For this review, take the finished solid that the model builds, in its own axes (mm). Give positions to 0.01 mm unless a question says otherwise; leave off trailing zeros. Loops run counter-clockwise (first coordinate to the right, second up) from the corner with the lowest first, then second, coordinate; pieces in that order, holes last. Notation, with made-up numbers: (45.25, -16) - (67.25, -16) arc R20 ccw to (67.25, 3) - close; hole circle Ø6 at (-38, 59). An arc over 180 degrees is marked (long way). Answer in a Markdown table with one row per item.
```python
from build123d import *

# Parameters (mm, degrees)
SKETCH1_W           = 42
SKETCH1_H           = 25
SKETCH1_R           = 1.5
BOSS_EXTRUDE1_DEPTH = 5


with BuildPart() as part:
    # Sketch1 → Boss-Extrude1 (new body)
    with BuildSketch(Plane.XY):
        with Locations((21, 12.5)):
            Rectangle(SKETCH1_W, SKETCH1_H)
        with Locations((10, 2.5)):
            Circle(SKETCH1_R, mode=Mode.SUBTRACT)
        with Locations((32, 2.5)):
            Circle(SKETCH1_R, mode=Mode.SUBTRACT)
    boss_extrude1 = extrude(amount=BOSS_EXTRUDE1_DEPTH)

    # Mirror1: Boss-Extrude1 across plane
    add(boss_extrude1.mirror(Plane(origin=(0, 25, 5), x_dir=(0, 0, 1), z_dir=(0, -1, 0))))


solid = part.part
```
1. Wall thickness on line 1 (Y direction, x = 32, z = 2.6): over which ranges is the line inside the solid? List them lowest first. Write a range as [from, to].
Values:
| item | result |
|---|---|
| line 1 | y = [0, 1], [4, 46], [49, 50] |
2. Mouldability with a two-part tool opening along Y and no side actions: class faces 1 (the face through (10, 49, 2)), 2 (the face through (21, 50, 2)), 3 (the face through (0, 25, 2)) as released by +Y, released by -Y, zero draft, split by the parting line, or undercut.
Values:
| item | result |
|---|---|
| face 1 | undercut |
| face 2 | released by +Y |
| face 3 | zero draft |
3. We need section A-A, the plane x = 32. Give the boundary of the cut face in (y, z), and give its area (3 significant figures).
Values:
| item | result |
|---|---|
| outline | (0, 0) - (1, 0) - (1, 5) - (0, 5) - close; (4, 0) - (46, 0) - (46, 5) - (4, 5) - close; (49, 0) - (50, 0) - (50, 5) - (49, 5) - close |
| area | 220 mm^2 |
4. Clearance check with a flat-ended pin moving along its axis: pin 1 (2.5 mm diameter, centred on x = 32, y = 2.5, fed in from +Z). State where the tip first meets the part, or that it passes through.
Values:
| item | result |
|---|---|
| pin 1 | passes through |
5. We need section B-B, the plane y = 47.5. Give the boundary of the cut face in (x, z), and give its area (3 significant figures).
Values:
| item | result |
|---|---|
| outline | (0, 0) - (8.5, 0) - (8.5, 5) - (0, 5) - close; (11.5, 0) - (30.5, 0) - (30.5, 5) - (11.5, 5) - close; (33.5, 0) - (42, 0) - (42, 5) - (33.5, 5) - close |
| area | 180 mm^2 |
